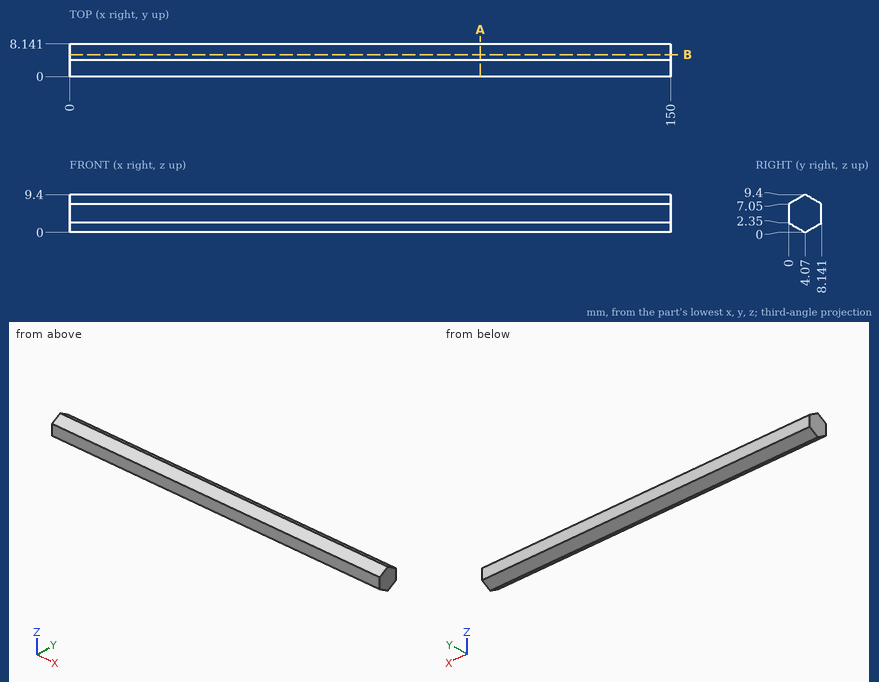
For this review, use the dimensioned drawing (mm, ordinates from the lowest corner) and the shaded views. Round coordinates to 2 decimals unless told otherwise and drop trailing zeros. Write each loop counter-clockwise with the first axis right and the second up, starting at its lowest first coordinate (ties: lowest second). Pieces come first, ordered by that corner, then holes. Notation, with made-up numbers: (38.25, 58.5) -> (43.25, 58.5) arc R10 ccw to (43.25, 71.5) -> close; hole circle Ø2 at (58.5, 27). An arc over 180 degrees is marked (long way). Use CSV: the item, a comma, the result in double quotes.
Q1. Consider section A-A (x = 102.5). Give the boundary of the cut face in (y, z).
Checks:
outline,"(0, 2.35) -> (4.07, 0) -> (8.14, 2.35) -> (8.14, 7.05) -> (4.07, 9.4) -> (0, 7.05) -> close"
Q2. To check wall thickness, follow probe 1 along Z at (x, y) = (86, 0.5); probe 2 along Z at (x, y) = (35, 7.25) (1 decimal); probe 3 along Y at (x, z) = (41, 9) (1 decimal). State the ranges of each line that lie inside material, in increasing order. Write a range as [from, to].
Checks:
probe 1,"[2.06, 7.34]"
probe 2,"[1.8, 7.6]"
probe 3,"[3.4, 4.8]"
Q3. For pin 1 Ø1.5 at (x, y) = (30, 5) entering from -Z, flat-tipped, find the tip position at first contact; note if it passes through.
Checks:
pin 1,"z = 0.1"
Q4. Consider section B-B (y = 5.5). Give the boundary of the cut face in (x, z) (1 decimal), then the cut area to 3 significant figures.
Checks:
outline,"(0, 0.8) -> (150, 0.8) -> (150, 8.6) -> (0, 8.6) -> close"
area,"1,160 mm²"
